Work out the finished part from the listing and answer in its coordinate system (mm). Face numbers are marked on the shaded views. A direction names the side the tool comes from. Round coordinates to 2 decimals unless told otherwise and drop trailing zeros. Write each loop counter-clockwise with the first axis right and the second up, starting at its lowest first coordinate (ties: lowest second). Pieces come first, ordered by that corner, then holes. Notation, with made-up numbers: (39, 53) - (66, 53) arc R8 cw to (66, 68) - close; hole circle Ø7 at (-10.5, 56.25). An arc over 180 degrees is marked (long way). Answer as a JSON object with one key per item and string values.
```python
from build123d import *

# Parameters (mm, degrees)
SKETCH_W        = 10
SKETCH_H        = 10
PAD_DEPTH       = 8
SKETCH001_R     = 1.85
POCKET_DEPTH    = 8
SKETCH002_R     = 2.75
POCKET001_DEPTH = 5
CHAMFER_SIZE    = 0.5


with BuildPart() as part:
    # Sketch → Pad (new body)
    with BuildSketch(Plane.XY):
        Rectangle(SKETCH_W, SKETCH_H)
    extrude(amount=PAD_DEPTH)

    # Sketch001 (on Face6 of Pad) → Pocket (cut)
    with BuildSketch(Plane.XY.offset(8)):
        Circle(SKETCH001_R)
    extrude(amount=-POCKET_DEPTH, mode=Mode.SUBTRACT)

    # Sketch002 (on Face5 of Pocket) → Pocket001 (cut)
    with BuildSketch(Plane.XY.offset(8)):
        Circle(SKETCH002_R)
    extrude(amount=-POCKET001_DEPTH, mode=Mode.SUBTRACT)

    # Chamfer
    chamfer_edges = [part.edges().sort_by_distance(p)[0] for p in [
        (-2.75, 0, 8),
    ]]
    chamfer(chamfer_edges, length=CHAMFER_SIZE)


solid = part.part
```
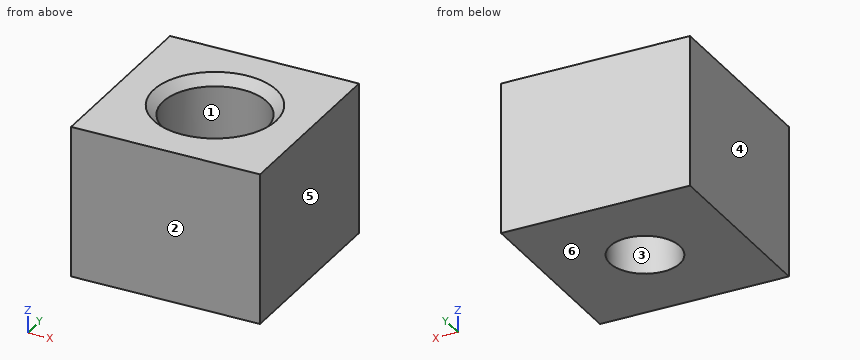
Item 1: A cutting plane is placed at C-C (z = 0.5). Write down the section's boundary in (x, y).
Results found:
{"outline": "(-5, -5) - (5, -5) - (5, 5) - (-5, 5) - close; hole circle Ø3.7 at (0, 0)"}
Item 2: A cutting plane is placed at D-D (z = 4). Write down the section's boundary in (x, y).
Results found:
{"outline": "(-5, -5) - (5, -5) - (5, 5) - (-5, 5) - close; hole circle Ø5.5 at (0, 0)"}
Item 3: For the marked faces 1 and 2, determine the directions among +Z, -Z, +X, -X, +Y, -Y from which every point of the face is accessible in a straight line to the end or side of a thin tool.
Results found:
{"face 1": "+Z", "face 2": "+Z, -Z, +X, -X, -Y"}
Item 4: This flat-tipped pin is pushed along its axis until it touches: P1, Ø5, axis at x = 0, y = 0, coming from the +Z side. Where does it stop, or does it pass through?
Results found:
{"P1": "z = 3"}
Item 5: Determine the mould class of the marked faces 3, 4, 5 and 6 for opening direction X: pulls with the +X half, pulls with the -X half, needs draft (parallel to the pull), parting line crosses it, or undercut.
Results found:
{"face 3": "undercut", "face 4": "pulls with the -X half", "face 5": "pulls with the +X half", "face 6": "needs draft"}
Item 6: A cutting plane is placed at A-A (x = 0). Write down the section's boundary in (y, z), and give its area (4 significant figures).
Results found:
{"outline": "(-5, 0) - (-1.85, 0) - (-1.85, 3) - (-2.75, 3) - (-2.75, 7.5) - (-3.25, 8) - (-5, 8) - close; (1.85, 0) - (5, 0) - (5, 8) - (3.25, 8) - (2.75, 7.5) - (2.75, 3) - (1.85, 3) - close", "area": "41.15 mm²"}
Item 7: Consider line 1 along Y through (x, z) = (0, 0.7); line 2 along Y through (x, z) = (0, 4.55); line 3 along Z through (x, y) = (1.75, -0.75). Determine where each line is inside the solid, lowest interval first.
Results found:
{"line 1": "-5 to -1.85, 1.85 to 5", "line 2": "-5 to -2.75, 2.75 to 5", "line 3": "0 to 3"}
